Drawing for the job (mm, zero at the part's lowest x, y, z). A direction names the side the tool comes from. Coordinates: 2 decimals unless noted, no trailing zeros. Write each loop counter-clockwise with the first axis right and the second up, starting at its lowest first coordinate (ties: lowest second). Pieces come first, ordered by that corner, then holes. Notation, with made-up numbers: (-28.5, 55) -> (6.5, 55) arc R9 ccw to (6.5, 70) -> close; hole circle Ø8 at (13, 78). An arc over 180 degrees is marked (long way). Answer as CSV lines item,"result". Start each with the question number.
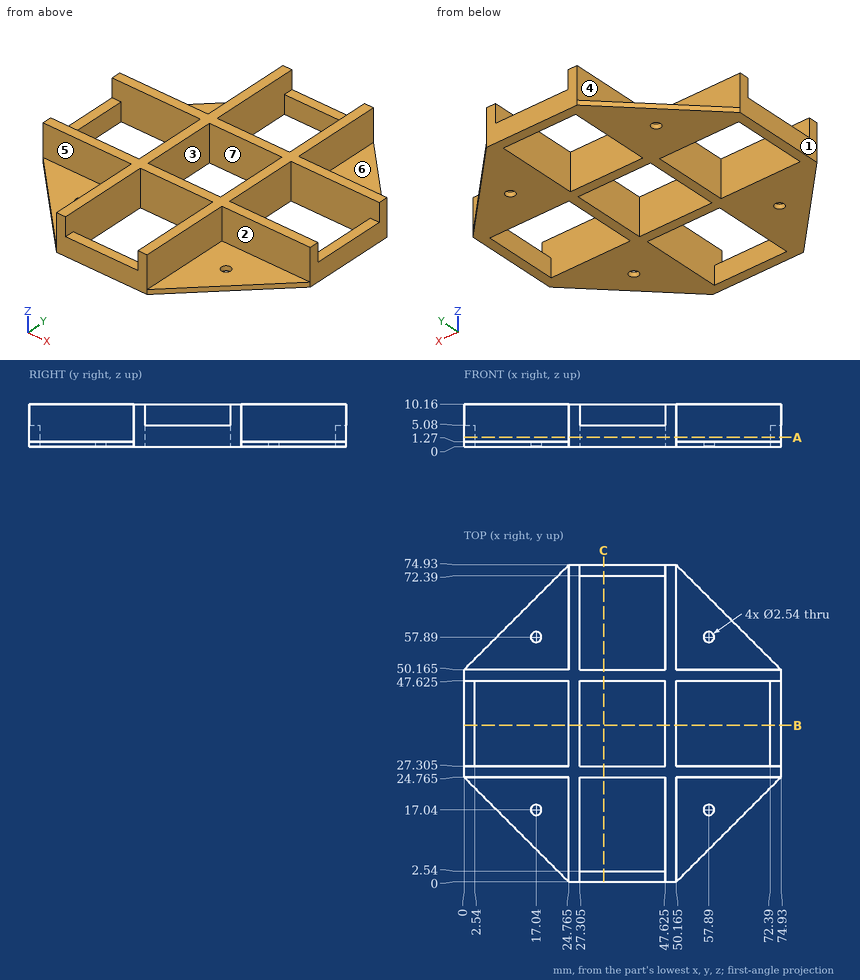
1. Cut at B-B (y = 37). Give the cut face in (x, z) (3 decimals), then the cut area to 3 significant figures.
2. Flat gauge pins, fed straight in: P1, Ø3, axis at x = 15.5, z = 6.5, coming from the +Y side (3 decimals); P2, Ø1.5, axis at y = 54.5, z = 8.5, coming from the +X side (3 decimals); P3, Ø5, axis at x = 58, z = 5, coming from the -Y side (3 decimals). Where does each tip first touch, or does it go through?
3. Wall check: line 1 (X direction, y = 35.5, z = 1.25) (3 decimals); line 2 (X direction, y = 5, z = 2) (3 decimals). Give the ranges that are in metal, low to high.
4. Mould opens along Y. For the marked faces 1, 2 and 3 say: pulls with the +Y half, pulls with the -Y half, needs draft (parallel to the pull), parting line crosses it, or undercut.
5. Cut at A-A (z = 2.25). Count the separate pieces of the cut face and the enclosed holes in it, then the cut area to 3 significant figures.
6. Tool access for the marked faces 4, 5, 6 and 7: list every direction of +Z, -Z, +X, -X, +Y, -Y with a clear straight run to the whole face (end or side of a thin tool).
Geometry check:
1,outline,"(0, 0) -> (2.54, 0) -> (2.54, 5.08) -> (0, 5.08) -> close; (24.765, 0) -> (27.305, 0) -> (27.305, 10.16) -> (24.765, 10.16) -> close; (47.625, 0) -> (50.165, 0) -> (50.165, 10.16) -> (47.625, 10.16) -> close; (72.39, 0) -> (74.93, 0) -> (74.93, 5.08) -> (72.39, 5.08) -> close"
1,area,"77.4 mm²"
2,P1,"y = 50.165"
2,P2,"x = 50.165"
2,P3,"y = 24.765"
3,line 1,"0 to 2.54, 24.765 to 27.305, 47.625 to 50.165, 72.39 to 74.93"
3,line 2,"24.765 to 27.305, 47.625 to 50.165"
4,face 1,"needs draft"
4,face 2,"pulls with the -Y half"
4,face 3,"undercut"
5,separate pieces,"1"
5,enclosed holes,"5"
5,area,"942 mm²"
6,face 4,"+Z, -X, +Y"
6,face 5,"+Z, -X, -Y"
6,face 6,"+Z, +X, +Y"
6,face 7,"+Z, -Z"
